Can you work these out from the model? Positions are in its coordinate system, mm. A direction names the side the tool comes from. Round coordinates to 2 decimals unless told otherwise and drop trailing zeros. Loops run counter-clockwise (first coordinate to the right, second up) from the corner with the lowest first, then second, coordinate; pieces in that order, holes last.
(1) Will these pins go through, and if not, where does the flat tip stop? pin 1 Ø5 at (x, y) = (27.5, 4) entering from -Z; pin 2 Ø1.5 at (x, y) = (69.5, -0.5) entering from +Z; pin 3 Ø3 at (y, z) = (0.5, 13.5) entering from -X; pin 4 Ø2.5 at (x, z) = (70.5, 11) entering from +Y.
(2) Thinking about a two-plate mould opening in X: for faces 1 (the face through (66.294, 0, -6)), 2 (the face through (4.12, 0.46, 6.47)), 3 (the face through (70, 5.08, 8)), which applies, released by +X, released by -X, zero draft, split by the parting line, or undercut?
(3) Which directions (+Z, -Z, +X, -X, +Y, -Y) give clear straight access to the entire face, cutting with the end or side of a thin tool? Please do faces 4 (the face through (10.16, 0, 0)), 5 (the face through (32.825, 10.074, -1.323)), 6 (the face through (69, 0, 4.826)).
(4) If I drill on line 1 along X through (y, z) = (-7, 8.25); line 2 along X through (y, z) = (2.75, -4.75); line 3 along Y through (x, z) = (-3, 1) (3 decimals), over which ranges is the centre line in solid material (lowest first)?
(5) I want a section at B-B on x = 29.5. Write out the boundary of the cut face in (y, z), plus the area to 3 significant figures.
(6) I want a section at D-D on z = -8. Write out the boundary of the cut face in (x, y).
(7) I want a section at A-A on z = 8.75. Write out the boundary of the cut face in (x, y) (3 decimals), plus the area to 3 significant figures.
(8) I want a section at C-C on y = -7. Write out the boundary of the cut face in (x, z).
from build123d import *

# Parameters (mm, degrees)
F0_W          = 5.842
F0_H          = 12.7
F0_R          = 3.175
F2_DEPTH      = 3.175
F3_R          = 1.524
F4_DEPTH      = 1.27
F4_DEPTH_BACK = 6.35
F5_DEPTH      = 56.134
F6_R          = 1.524
F7_DEPTH      = 17.78
F8_DEPTH      = 10.414


with BuildPart() as f1:
    # F0 (on Front) → F1 (revolve)
    with BuildSketch(Plane.XZ):
        Polygon((5.842, 12.7), (5.842, 0), (66.294, 0), (66.294, 12.7), (56.134, 12.7), (56.134, 10.16), (10.16, 10.16), (10.16, 12.7), align=None)
        with Locations((2.921, 6.35)):
            Rectangle(F0_W, F0_H)
    revolve(axis=Axis((33.147, 0, 0), (-1, 0, 0)))

    # F0 (on Front) → F2 (join, symmetric)
    with BuildSketch(Plane.XZ):
        with BuildLine():
            Line((-0.9398, 0), (0, 0))
            Line((0, 0), (0, 12.7))
            Line((0, 12.7), (5.842, 12.7))
            Line((5.842, 12.7), (5.842, 15.24))
            Line((5.842, 15.24), (-0.508, 15.24))
            Line((-0.508, 15.24), (-10.8806298187, 3.8475430269))
            ThreePointArc((-10.8806298187, 3.8475430269), (-4.5919612295, 5.3297205562), (-0.9398, 0))
        make_face()
        with BuildLine():
            ThreePointArc((-8.1826630726, -5.5069827884), (-3.1957909266, -4.5493385486), (-0.9398, 0))
            ThreePointArc((-0.9398, 0), (-4.5919612295, 5.3297205562), (-10.8806298187, 3.8475430269))
            ThreePointArc((-10.8806298187, 3.8475430269), (-12.1459778134, -1.5837270034), (-8.1826630726, -5.5069827884))
        make_face()
        with Locations((-6.6548, 0)):
            Circle(F0_R, mode=Mode.SUBTRACT)
        with Locations((2.921, 6.35)):
            Rectangle(F0_W, F0_H)
    extrude(amount=F2_DEPTH, both=True)

    # F3 (on face) → F4 (join, two sides)
    with BuildSketch(Plane.YZ.offset(66.294)) as f4_sk:
        with BuildLine():
            ThreePointArc((-5.08, 0), (0, -5.08), (5.08, 0))
            ThreePointArc((5.08, 0), (0, 5.08), (-5.08, 0))
        make_face()
        Circle(F3_R, mode=Mode.SUBTRACT)
        with BuildLine():
            ThreePointArc((-5.08, 0), (0, 5.08), (5.08, 0))
            Line((5.08, 0), (5.08, 15.24))
            Line((5.08, 15.24), (-5.08, 15.24))
            Line((-5.08, 15.24), (-5.08, 0))
        make_face()
    extrude(amount=-F4_DEPTH)
    extrude(f4_sk.sketch, amount=F4_DEPTH_BACK)

    # F3 (on face) → F5 (cut, through all)
    with BuildSketch(Plane.YZ.offset(66.294)):
        Circle(F3_R)
    extrude(amount=-F5_DEPTH, mode=Mode.SUBTRACT)

    # F6 (on face) → F7 (cut)
    with BuildSketch(Plane.XY.offset(15.24)):
        with Locations((2.667, 0)):
            Circle(F6_R)
    extrude(amount=-F7_DEPTH, mode=Mode.SUBTRACT)

    # F6 (on face) → F8 (cut)
    with BuildSketch(Plane.XY.offset(15.24)):
        with Locations((68.834, 0)):
            Circle(F6_R)
    extrude(amount=-F8_DEPTH, mode=Mode.SUBTRACT)


solid = f1.part
Filled sheet:
1. pin 1: stops at z = -10.05
1. pin 2: stops at z = 15.24
1. pin 3: stops at x = -3.46
1. pin 4: stops at y = 5.08
2. face 1: released by +X
2. face 2: undercut
2. face 3: zero draft
3. face 4: +X
3. face 5: none
3. face 6: +Z
4. line 1: x = 0 to 10.16, 56.13 to 66.29
4. line 2: x = -9.83 to -3.48, 0 to 66.29
4. line 3: y = -3.175 to 3.175
5. outline: circle Ø20.32 at (0, 0); hole circle Ø3.05 at (0, 0)
5. area: 317 mm2
6. outline: (0, -9.86) - (10.16, -9.86) - (10.16, -6.26) - (56.13, -6.26) - (56.13, -9.86) - (66.29, -9.86) - (66.29, 9.86) - (56.13, 9.86) - (56.13, 6.26) - (10.16, 6.26) - (10.16, 9.86) - (0, 9.86) - close
7. outline: (-6.417, -3.175) - (0, -3.175) - (0, -9.205) - (10.16, -9.205) - (10.16, -5.164) - (56.134, -5.164) - (56.134, -9.205) - (66.294, -9.205) - (66.294, -5.08) - (72.644, -5.08) - (72.644, 5.08) - (66.294, 5.08) - (66.294, 9.205) - (56.134, 9.205) - (56.134, 5.164) - (10.16, 5.164) - (10.16, 9.205) - (0, 9.205) - (0, 3.175) - (-6.417, 3.175) - close; hole circle Ø3.048 at (2.667, 0); hole circle Ø3.048 at (68.834, 0)
7. area: 940 mm2
8. outline: (0, -10.6) - (10.16, -10.6) - (10.16, -7.36) - (56.13, -7.36) - (56.13, -10.6) - (66.29, -10.6) - (66.29, 10.6) - (56.13, 10.6) - (56.13, 7.36) - (10.16, 7.36) - (10.16, 10.6) - (0, 10.6) - close
